Autodesk Inventor part; units mm, degrees
ref_plane "YZ Plane" through (0, 0, 0) normal (1, 0, 0) x (0, 1, 0)
ref_plane "XZ Plane" through (0, 0, 0) normal (0, 1, 0) x (-1, 0, 0)
ref_plane "XY Plane" through (0, 0, 0) normal (0, 0, 1) x (1, 0, 0)
sketch "Sketch1" plane through (0, 0, 0) normal (0, 0, 1) x (1, 0, 0)
  line L0 (12.7, -12.7) -> (-12.7, -12.7)
  line L1 (-12.7, -12.7) -> (-12.7, 12.7)
  line L2 (-12.7, 12.7) -> (5.08, 12.7)
  line L3 (12.7, 5.08) -> (12.7, -12.7)
  line L4 (12.7, -12.7) -> (-12.7, 12.7) construction
  line L5 (-12.7, -12.7) -> (12.7, 12.7) construction
  line L6 (5.08, 12.7) -> (12.7, 5.08)
  point P0 (0, 0)
  dimension "d0" = 25.4
  dimension "d1" = 25.4
  dimension "d2" = 7.62
  dimension "d3" = 7.62
extrude "Extrusion1" add sketch "Sketch1" along normal mid plane 273.05
equation "\"d3\" = d2"
properties part number "Shooter Base Cleat"
Here's how the part is built. I have some questions about the finished solid (model axes, mm). Give positions to 0.01 mm unless a question says otherwise; leave off trailing zeros. Loops run counter-clockwise (first coordinate to the right, second up) from the corner with the lowest first, then second, coordinate; pieces in that order, holes last. Notation, with made-up numbers: M -33.5,-37 L -15.5,-37 A31 cw -15.5,-13 Z; hole C 29,86 d1. An arc over 180 degrees is marked long. Use one line per item in the form item = value. Start each with the question number.
Q1. If we section it at B-B (x = 10.25): Write out the boundary of the cut face in (y, z) (3 decimals), then the cut area to 3 significant figures.
Q2. I need wall thicknesses on line 1 along Y through (x, z) = (9.5, -38); line 2 along Y through (x, z) = (11, 122). Which ranges of each line are inside material? Lowest first, please.
Q3. If we section it at A-A (z = 7.5): Write out the boundary of the cut face in (x, y).
Taken from the geometry:
q1.outline = M -12.7,-136.525 L 7.53,-136.525 L 7.53,136.525 L -12.7,136.525 Z
q1.area = 5,520 mm^2
q2.line_1 = -12.7 to 8.28
q2.line_2 = -12.7 to 6.78
q3.outline = M -12.7,-12.7 L 12.7,-12.7 L 12.7,5.08 L 5.08,12.7 L -12.7,12.7 Z
